Verification items for the finished model (mm, model axes). A direction names the side the tool comes from. Give positions to 0.01 mm unless a question says otherwise; leave off trailing zeros. Loops run counter-clockwise (first coordinate to the right, second up) from the corner with the lowest first, then second, coordinate; pieces in that order, holes last. Notation, with made-up numbers: M -25.75,27.25 L 30.25,27.25 A34 cw 30.25,65.25 Z; hole C 79.5,-25.75 d6. An arc over 180 degrees is marked long. Write each question's results on one line, items separated by ' | '. Start each with the question number.
```python
from build123d import *

# Parameters (mm, degrees)
F1_DEPTH = 20
F3_DEPTH = 25
F5_DEPTH = 50
F7_DEPTH = 40


with BuildPart() as f1:
    # F0 (on Top) → F1 (new body)
    with BuildSketch(Plane.XY):
        with BuildLine():
            ThreePointArc((2, 16.8819430161), (-7.8722441486, 15.0674407935), (-15, 8))
            Line((-15, 8), (-15, 1.73e-08))
            Line((-15, 1.73e-08), (-15, -8))
            ThreePointArc((-15, -8), (-2.5191792462, -16.8123090599), (11.9964033105, -12.0451777742))
            Line((11.9964033105, -12.0451777742), (2, 0.6911440225))
            Line((2, 0.6911440225), (2, 16.8819430161))
        make_face()
        with BuildLine():
            ThreePointArc((9.2611890072, -11.7995922884), (-6.5605702914, -13.4892148568), (-15, 1.73e-08))
            ThreePointArc((-15, 1.73e-08), (-10.6066017117, 10.6066017239), (0, 15))
            Line((0, 15), (0, 0))
            Line((0, 0), (9.2611890072, -11.7995922884))
        make_face(mode=Mode.SUBTRACT)
        with BuildLine():
            Line((-15, 1.73e-08), (-15, 8))
            ThreePointArc((-15, 8), (-17, 0), (-15, -8))
            Line((-15, -8), (-15, 1.73e-08))
        make_face()
    extrude(amount=F1_DEPTH)

    # F2 (on Top) → F3 (join)
    with BuildSketch(Plane.XY):
        with BuildLine():
            Line((-12.2984962158, 1.5833490395), (0, 0))
            Line((0, 0), (0, 1.7140309842))
            Line((0, 1.7140309842), (-10.2605423337, 3.0350071071))
            ThreePointArc((-10.2605423337, 3.0350071071), (-6.4037263169, 8.5721809582), (0, 10.6999998655))
            Line((0, 10.6999998655), (0, 12.4000001351))
            ThreePointArc((0, 12.4000001351), (-8.1892147074, 9.3111098064), (-12.2984962158, 1.5833490395))
        make_face()
    extrude(amount=F3_DEPTH)

    # F4 (on Top) → F5 (join)
    with BuildSketch(Plane.XY):
        with BuildLine():
            Line((4.6733382454, -2.7149306533), (5.8758648402, -4.2470582801))
            ThreePointArc((5.8758648402, -4.2470582801), (6.8524321368, 2.3680087553), (2, 6.968736733))
            Line((2, 6.968736733), (2, 5.0210495724))
            ThreePointArc((2, 5.0210495724), (5.1082979893, 1.7652848101), (4.6733382454, -2.7149306533))
        make_face()
    extrude(amount=F5_DEPTH)

    # F2 (on Top) + F6 (on Top) → F7 (join)
    with BuildSketch(Plane.XY):
        with BuildLine():
            Line((-12.2984962158, 1.5833490395), (0, 0))
            Line((0, 0), (0, 1.7140309842))
            Line((0, 1.7140309842), (-10.2605423337, 3.0350071071))
            ThreePointArc((-10.2605423337, 3.0350071071), (-6.4037263169, 8.5721809582), (0, 10.6999998655))
            Line((0, 10.6999998655), (0, 12.4000001351))
            ThreePointArc((0, 12.4000001351), (-8.1892147074, 9.3111098064), (-12.2984962158, 1.5833490395))
        make_face()
    with BuildSketch(Plane.XY):
        with BuildLine():
            ThreePointArc((-9.3527705449, 1.2041065834), (-4.6584728249, -8.1989524008), (5.8221775641, -7.4179807186))
            Line((5.8221775641, -7.4179807186), (4.4831560663, -5.7119462422))
            ThreePointArc((4.4831560663, -5.7119462422), (-3.5870875587, -6.3133050802), (-7.2017607749, 0.9271784782))
            Line((-7.2017607749, 0.9271784782), (-9.3527705449, 1.2041065834))
        make_face()
    extrude(amount=F7_DEPTH)


solid = f1.part
```
1. Set-up check for faces 1 (the face through (5.266, -3.47, 34.79)), 2 (the face through (2, 12, 10)), 3 (the face through (2, 6, 35)), 4 (the face through (2, 3, 10)): record each of +Z, -Z, +X, -X, +Y, -Y from which the full face is reachable in a straight line by a thin tool's end or side.
2. Section check B-B, the plane y = -1. Record the boundary of the cut face in (x, z).
3. Section check D-D, the plane z = 13. Record the boundary of the cut face in (x, y) (1 decimal).
4. Thickness scan on probe 1 along X at (y, z) = (-7.5, 13.5); probe 2 along Y at (x, z) = (-8, 3.5); probe 3 along Y at (x, z) = (-11.25, 18). Record the ranges inside material, lowest first.
5. Section check C-C, the plane x = -13.5. Record the boundary of the cut face in (y, z).
6. Section check A-A, the plane z = 31. Record the boundary of the cut face in (x, y) (1 decimal), plus the area to 3 significant figures.
7. Depth check by flat-ended pin: pin 1 Ø12 at (x, y) = (-6, -2.5) entering from +Z; pin 2 Ø8 at (x, z) = (7.5, 17) entering from +Y; pin 3 Ø1.3 at (y, z) = (4, 8) entering from +X; pin 4 Ø1 at (y, z) = (13, 36) entering from -X. Enter the tip coordinate at first touch or a pass-through.
Filled sheet:
1) face 1: +Z | face 2: +Z, -Z, +X, +Y | face 3: +Z, +Y | face 4: +Z, -Z
2) outline: M -16.97,0 L -14.97,0 L -14.97,20 L -16.97,20 Z; M -9.38,0 L -7.19,0 L -7.19,40 L -9.38,40 Z; M 0.78,0 L 3.33,0 L 3.33,20 L 0.78,20 Z; M 5.31,0 L 7.18,0 L 7.18,50 L 5.31,50 Z
3) outline: M 2,7 L 2,16.9 A17 ccw long 12,-12 L 5.9,-4.2 A7.3 ccw Z; hole M -12.3,1.6 A12.4 cw 0,12.4 L 0,15 A15 ccw long 9.3,-11.8 L 5.8,-7.4 A9.4 cw -9.4,1.2 Z; hole M -10.3,3 L 0,1.7 L 0,10.7 A10.7 ccw Z; hole M -7.2,0.9 A7.3 ccw 4.5,-5.7 L 0,0 Z; hole M 2,0.7 L 4.7,-2.7 A5.4 ccw 2,5 Z
4) probe 1: -15.26 to -12.99, -5.72 to 5.72, 5.89 to 8.43 | probe 2: -15 to -12.69, -4.99 to 2.74, 7.11 to 9.47, 12.69 to 15 | probe 3: -12.75 to -9.92, 1.45 to 5.22, 9.92 to 12.75
5) outline: M -10.33,0 L -6.54,0 L -6.54,20 L -10.33,20 Z; M 6.54,0 L 10.33,0 L 10.33,20 L 6.54,20 Z
6) outline: M -12.3,1.6 L -9.4,1.2 A9.4 ccw 5.8,-7.4 L 4.5,-5.7 A7.3 cw -7.2,0.9 L 0,0 L 0,1.7 L -10.3,3 A10.7 cw 0,10.7 L 0,12.4 A12.4 ccw Z; M 2,5 A5.4 cw 4.7,-2.7 L 5.9,-4.2 A7.3 ccw 2,7 Z | area: 110 mm2
7) pin 1: z = 40 | pin 2: y = 6.35 | pin 3: x = 6.43 | pin 4: through
